The drawing under review shows one solid part. Ordinate dimensions are in mm from its lowest x, y, z. A direction names the side the tool comes from. Coordinates: 2 decimals unless noted, no trailing zeros. Write each loop counter-clockwise with the first axis right and the second up, starting at its lowest first coordinate (ties: lowest second). Pieces come first, ordered by that corner, then holes. Notation, with made-up numbers: (53, 81) - (91, 81) arc R8 ccw to (91, 95) - close; hole circle Ø3 at (-0.75, 43). An arc over 180 degrees is marked (long way). Put each result on its own line as item: value. Start each with the question number.
Item 1: To check wall thickness, follow L1, parallel to X at y = 1.45, z = 12.7 (1 decimal); L2, parallel to Z at x = 25, y = 3 (1 decimal); L3, parallel to Y at x = 25, z = 24. State the ranges of each line that lie inside material, in increasing order. Write a range as [from, to].
Item 2: Mouldability with a two-part tool opening along Z and no side actions: class the marked faces 4, 5 and 6 as pulls with the +Z half, pulls with the -Z half, needs draft (parallel to the pull), parting line crosses it, or undercut.
Item 3: Consider section B-B on x = 25. Give the boundary of the cut face in (y, z) (1 decimal).
Item 4: Consider section D-D on y = 20. Give the boundary of the cut face in (x, z), then the cut area to 3 significant figures.
Item 5: For pin 1 (3.5 mm diameter, centred on x = 10, y = 43.13, fed in from -Z); pin 2 (5 mm diameter, centred on x = 40, y = 13.13, fed in from -Z); pin 3 (17 mm diameter, centred on x = 25.5, z = 14.5, fed in from +Y); pin 4 (8.5 mm diameter, centred on x = 25, z = 38.1, fed in from +Y), all flat-tipped, find the tip position at first contact; note any pin that passes through.
Item 6: Consider section C-C on x = 9. Give the boundary of the cut face in (y, z) (1 decimal).
Item 7: Machinability: for the marked faces 1, 2 and 3, which of the approach directions +Z, -Z, +X, -X, +Y, -Y give a long, thin tool a straight path to every point of the face, cutting with its end or side? Answer none if there is none.
Item 8: Consider section A-A on z = 38.1. Give the boundary of the cut face in (x, y) (1 decimal), then the cut area to 3 significant figures.
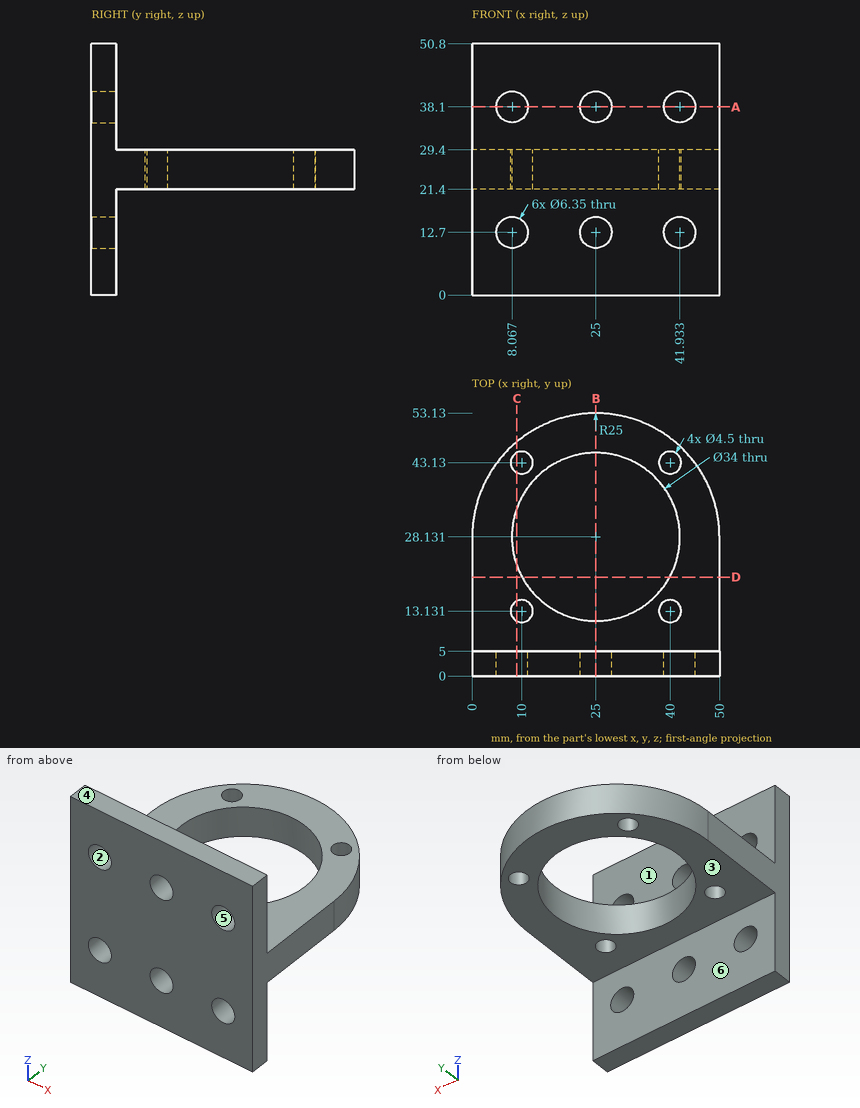
Report:
1. L1: [0, 4.9], [11.2, 21.8], [28.2, 38.8], [45.1, 50]
1. L2: [0, 9.5], [15.9, 34.9], [41.3, 50.8]
1. L3: [0, 11.13], [45.13, 53.13]
2. face 4: pulls with the +Z half
2. face 5: undercut
2. face 6: needs draft
3. outline: (0, 0) - (5, 0) - (5, 9.5) - (0, 9.5) - close; (0, 15.9) - (5, 15.9) - (5, 21.4) - (11.1, 21.4) - (11.1, 29.4) - (5, 29.4) - (5, 34.9) - (0, 34.9) - close; (0, 41.3) - (5, 41.3) - (5, 50.8) - (0, 50.8) - close; (45.1, 21.4) - (53.1, 21.4) - (53.1, 29.4) - (45.1, 29.4) - close
4. outline: (0, 21.4) - (10.07, 21.4) - (10.07, 29.4) - (0, 29.4) - close; (39.93, 21.4) - (50, 21.4) - (50, 29.4) - (39.93, 29.4) - close
4. area: 161 mm²
5. pin 1: through
5. pin 2: z = 21.4
5. pin 3: y = 53.13
5. pin 4: y = 5
6. outline: (0, 0) - (5, 0) - (5, 9.7) - (0, 9.7) - close; (0, 15.7) - (5, 15.7) - (5, 21.4) - (11.1, 21.4) - (11.1, 29.4) - (5, 29.4) - (5, 35.1) - (0, 35.1) - close; (0, 41.1) - (5, 41.1) - (5, 50.8) - (0, 50.8) - close; (15.1, 21.4) - (22.4, 21.4) - (22.4, 29.4) - (15.1, 29.4) - close; (33.9, 21.4) - (41.1, 21.4) - (41.1, 29.4) - (33.9, 29.4) - close; (45.1, 21.4) - (47.3, 21.4) - (47.3, 29.4) - (45.1, 29.4) - close
7. face 1: +Z, +X, -X, +Y
7. face 2: +Y, -Y
7. face 3: -Z, +X, -X, +Y
8. outline: (0, 0) - (4.9, 0) - (4.9, 5) - (0, 5) - close; (11.2, 0) - (21.8, 0) - (21.8, 5) - (11.2, 5) - close; (28.2, 0) - (38.8, 0) - (38.8, 5) - (28.2, 5) - close; (45.1, 0) - (50, 0) - (50, 5) - (45.1, 5) - close
8. area: 155 mm²
